Model file for the job. Use its own axes, mm. A direction names the side the tool comes from. Coordinates: 2 decimals unless noted, no trailing zeros. Order: outer loops, then holes, each group sorted by start corner. A loop starts at its lowest first (then second) coordinate and runs counter-clockwise, first axis right, second up. Notation, with made-up numbers: (50.5, 51) -> (59.5, 51) arc R21 cw to (59.5, 87) -> close; hole circle Ø5 at (2.5, -20). An arc over 180 degrees is marked (long way). Return JSON: item names as keys, results as strings. Group by question number.
1) Cut at B-B (z = -102.5). Write the cut outline in (x, y), and give its area (3 significant figures).
2) Flat gauge pins, fed straight in: pin 1 (9.5 mm diameter, centred on y = 172, z = 267.5, fed in from +X); pin 2 (2 mm diameter, centred on x = 152.5, y = 166.5, fed in from -Z); pin 3 (5 mm diameter, centred on y = 247.12, z = -31.83, fed in from -X). Where does each tip first touch, or does it go through?
3) Cut at A-A (x = 2). Write the cut outline in (y, z), and give its area (3 significant figures).
4) Pull direction X, two halves, no side cores. Call faces 5 (the flat face through (150, 101, 328)), 6 (the cylindrical face through (199.014, 138.708, 247.599)), 7 (the flat face through (148, 103, 326)): +X half, -X half, draft (parallel to the pull), parting line (faces both ways), or undercut.
5) Probe line 1 (Y direction, x = 14.5, z = -236.95); line 2 (Y direction, x = 14, z = -237); line 3 (Z direction, x = -135.5, y = 55). List the from-to ranges inside material, lowest first.
6) Which spindle directions (+Z, -Z, +X, -X, +Y, -Y) get a long thin tool onto all of the face, cutting with end or side? Do faces 1 (the flat face through (198, 140, 31)), 2 (the cylindrical face through (-199.01, 231.29, -94.59)), 3 (the flat face through (175, 101, 292.174)), 4 (the flat face through (149.081, 171.234, 320.121)). Say none if no direction does.
from build123d import *

# Parameters (mm, degrees)
BOSS_EXTRUDE1_DEPTH     = 1.5
BOSS_EXTRUDE2_DEPTH     = 280
SKETCH4_W               = 400
SKETCH4_H               = 42.385541564
BOSS_EXTRUDE3_DEPTH     = 2
CUT_EXTRUDE1_DEPTH      = 609.61485268
CUT_EXTRUDE1_DEPTH_BACK = 609.61485268
SKETCH8_R               = 4.39
SKETCH8_R_2             = 2.39
BOSS_EXTRUDE5_DEPTH     = 15
SKETCH10_R              = 3
CUT_EXTRUDE2_DEPTH      = 2
SKETCH5_R               = 2
SKETCH5_R_2             = 10
CUT_EXTRUDE7_DEPTH      = 2
SKETCH21_W              = 300
SKETCH21_H              = 1.5
BOSS_EXTRUDE9_DEPTH     = 10
SKETCH22_W              = 300
SKETCH22_H              = 1.5
BOSS_EXTRUDE10_DEPTH    = 10
BOSS_EXTRUDE11_DEPTH    = 0.75
BOSS_EXTRUDE12_DEPTH    = 0.75
BOSS_EXTRUDE13_DEPTH    = 0.75
BOSS_EXTRUDE14_DEPTH    = 0.75
SKETCH27_W              = 200
SKETCH27_H              = 1.5
BOSS_EXTRUDE15_DEPTH    = 10
BOSS_EXTRUDE16_DEPTH    = 0.75
BOSS_EXTRUDE17_DEPTH    = 0.75
SKETCH30_R              = 24
SKETCH30_R_2            = 1.5
CUT_EXTRUDE8_DEPTH      = 2
SKETCH33_R              = 2
CUT_EXTRUDE9_DEPTH      = 2
SKETCH42_W              = 340
SKETCH42_H              = 12
SKETCH42_R              = 1.6
CUT_EXTRUDE13_DEPTH     = 40


with BuildPart() as part:
    # Sketch1 → Boss-Extrude1 (new body)
    with BuildSketch(Plane(origin=(0, 0, 0), x_dir=(1, 0, 0), z_dir=(0, 1, 0))):
        Polygon((-200, 237.826300096), (200, 237.826300096), (200, -292.173699904), (150, -292.173699904), (150, -362.173699904), (-200, -362.173699904), align=None)
    extrude(amount=BOSS_EXTRUDE1_DEPTH)

    # Sketch2 → Boss-Extrude2 (add)
    with BuildSketch(Plane(origin=(0, 1.5, 0), x_dir=(1, 0, 0), z_dir=(0, 1, 0))):
        Polygon((-200, 237.826300096), (-200, -362.173699904), (150, -362.173699904), (150, -292.173699904), (200, -292.173699904), (200, 237.826300096), align=None)
        Polygon((-198, 235.826300096), (-198, -360.173699904), (148, -360.173699904), (148, -290.173699904), (198, -290.173699904), (198, 235.826300096), align=None, mode=Mode.SUBTRACT)
    extrude(amount=BOSS_EXTRUDE2_DEPTH)

    # Sketch4 → Boss-Extrude3 (add)
    with BuildSketch(Plane(origin=(0, 0, -237.826300096), x_dir=(-1, 0, 0), z_dir=(0, 0, -1))):
        with Locations((0, 213.483316708)):
            Rectangle(SKETCH4_W, SKETCH4_H)
    extrude(amount=-BOSS_EXTRUDE3_DEPTH)

    # Sketch3 → Cut-Extrude1 (cut, two sides: drawn at the far end of the back side and taken through both)
    with BuildSketch(Plane.ZY.offset(200).offset(-CUT_EXTRUDE1_DEPTH_BACK)):
        Polygon((362.173699904, 121.117558148), (227.596852099, 281.5), (362.173699904, 281.5), align=None)
    extrude(amount=CUT_EXTRUDE1_DEPTH + CUT_EXTRUDE1_DEPTH_BACK, mode=Mode.SUBTRACT)

    # Sketch8 → Boss-Extrude5 (add)
    # profile 1 of 2: a face of its own
    with BuildSketch(Plane(origin=(-198, 0, 0), x_dir=(0, 0, -1), z_dir=(1, 0, 0))):
        with Locations((-265.673697326, 172.19919718)):
            Circle(SKETCH8_R)
        with Locations((-265.673697326, 172.19919718)):
            Circle(SKETCH8_R_2, mode=Mode.SUBTRACT)
    # profile 2 of 2: a face of its own
    with BuildSketch(Plane(origin=(-198, 0, 0), x_dir=(0, 0, -1), z_dir=(1, 0, 0))):
        with Locations((-265.173699904, 16.5)):
            Circle(SKETCH8_R)
        with Locations((-265.173699904, 16.5)):
            Circle(SKETCH8_R_2, mode=Mode.SUBTRACT)
    extrude(amount=BOSS_EXTRUDE5_DEPTH)

    # Sketch10 → Cut-Extrude2 (cut)
    with BuildSketch(Plane.ZY.offset(-148)):
        with BuildLine():
            Line((333.923699904, 90.5), (319.923699904, 90.5))
            Line((319.923699904, 90.5), (319.923699904, 87.5))
            Line((319.923699904, 87.5), (315.673699904, 87.5))
            ThreePointArc((315.673699904, 87.5), (304.673699904, 76.5), (315.673699904, 65.5))
            Line((315.673699904, 65.5), (338.173699904, 65.5))
            ThreePointArc((338.173699904, 65.5), (349.173699904, 76.5), (338.173699904, 87.5))
            Line((338.173699904, 87.5), (333.923699904, 87.5))
            Line((333.923699904, 87.5), (333.923699904, 90.5))
        make_face()
        with Locations((300.973699904, 103.45)):
            Circle(SKETCH10_R)
        with Locations((352.873699904, 103.45)):
            Circle(SKETCH10_R)
        with Locations((300.973699904, 49.55)):
            Circle(SKETCH10_R)
        with Locations((352.873699904, 49.55)):
            Circle(SKETCH10_R)
    extrude(amount=-CUT_EXTRUDE2_DEPTH, mode=Mode.SUBTRACT)

    # Sketch5 → Cut-Extrude7 (cut)
    with BuildSketch(Plane.ZY.offset(200)):
        with Locations((-115.826300096, 247.120648807)):
            Circle(SKETCH5_R)
        with Locations((-116.326300096, 223.125857706)):
            Circle(SKETCH5_R)
        with Locations((-91.826300096, 223.120648807)):
            Circle(SKETCH5_R)
        with Locations((-91.826300096, 247.120648807)):
            Circle(SKETCH5_R)
        with Locations((-103.826300096, 235.120648807)):
            Circle(SKETCH5_R_2)
        with Locations((-55.826300096, 247.120648807)):
            Circle(SKETCH5_R)
        with Locations((-56.326300096, 223.125857706)):
            Circle(SKETCH5_R)
        with Locations((-31.826300096, 223.120648807)):
            Circle(SKETCH5_R)
        with Locations((-31.826300096, 247.120648807)):
            Circle(SKETCH5_R)
        with Locations((-43.826300096, 235.120648807)):
            Circle(SKETCH5_R_2)
        with Locations((4.173699904, 247.120648807)):
            Circle(SKETCH5_R)
        with Locations((3.673699904, 223.125857706)):
            Circle(SKETCH5_R)
        with Locations((28.173699904, 223.120648807)):
            Circle(SKETCH5_R)
        with Locations((28.173699904, 247.120648807)):
            Circle(SKETCH5_R)
        with Locations((16.173699904, 235.120648807)):
            Circle(SKETCH5_R_2)
        with Locations((64.173699904, 247.120648807)):
            Circle(SKETCH5_R)
        with Locations((63.673699904, 223.125857706)):
            Circle(SKETCH5_R)
        with Locations((88.173699904, 223.120648807)):
            Circle(SKETCH5_R)
        with Locations((88.173699904, 247.120648807)):
            Circle(SKETCH5_R)
        with Locations((76.173699904, 235.120648807)):
            Circle(SKETCH5_R_2)
    extrude(amount=-CUT_EXTRUDE7_DEPTH, mode=Mode.SUBTRACT)

    # Sketch21 → Boss-Extrude9 (add)
    with BuildSketch(Plane(origin=(0, 0, -237.826300096), x_dir=(-1, 0, 0), z_dir=(0, 0, -1))):
        with Locations((0, 270.75)):
            Rectangle(SKETCH21_W, SKETCH21_H)
    extrude(amount=BOSS_EXTRUDE9_DEPTH)

    # Sketch22 → Boss-Extrude10 (add)
    with BuildSketch(Plane.ZY.offset(200)):
        with Locations((-7.826300096, 270.75)):
            Rectangle(SKETCH22_W, SKETCH22_H)
    boss_extrude10 = extrude(amount=BOSS_EXTRUDE10_DEPTH)

    # Sketch23 → Boss-Extrude11 (add, symmetric)
    with BuildSketch(Plane(origin=(0, 0, -77.826300096), x_dir=(-1, 0, 0), z_dir=(0, 0, -1))):
        Polygon((210, 270), (200, 270), (200, 260), align=None)
    boss_extrude11 = extrude(amount=BOSS_EXTRUDE11_DEPTH, both=True)

    # Sketch24 → Boss-Extrude12 (add, symmetric)
    with BuildSketch(Plane.XY.offset(52.173699904)):
        Polygon((-210, 270), (-200, 260), (-200, 270), align=None)
    boss_extrude12 = extrude(amount=BOSS_EXTRUDE12_DEPTH, both=True)

    # Sketch25 → Boss-Extrude13 (add, symmetric)
    with BuildSketch(Plane(origin=(100, 0, 0), x_dir=(0, 0, -1), z_dir=(1, 0, 0))):
        Polygon((247.826300096, 270), (237.826300096, 270), (237.826300096, 260), align=None)
    extrude(amount=BOSS_EXTRUDE13_DEPTH, both=True)

    # Sketch26 → Boss-Extrude14 (add, symmetric)
    with BuildSketch(Plane.ZY.offset(100)):
        Polygon((-247.826300096, 270), (-237.826300096, 260), (-237.826300096, 270), align=None)
    extrude(amount=BOSS_EXTRUDE14_DEPTH, both=True)

    # Mirror1: Boss-Extrude10, Boss-Extrude11, Boss-Extrude12 across plane
    add(boss_extrude10.mirror(Plane(origin=(0, 0, 0), x_dir=(0, 0, 1), z_dir=(1, 0, 0))))
    add(boss_extrude11.mirror(Plane(origin=(0, 0, 0), x_dir=(0, 0, 1), z_dir=(1, 0, 0))))
    add(boss_extrude12.mirror(Plane(origin=(0, 0, 0), x_dir=(0, 0, 1), z_dir=(1, 0, 0))))

    # Sketch27 → Boss-Extrude15 (add)
    with BuildSketch(Plane.XY.offset(362.173699904)):
        with Locations((-25, 110.367558148)):
            Rectangle(SKETCH27_W, SKETCH27_H)
    extrude(amount=BOSS_EXTRUDE15_DEPTH)

    # Sketch28 → Boss-Extrude16 (add, symmetric)
    with BuildSketch(Plane.ZY.offset(95)):
        Polygon((372.173699904, 109.617558148), (362.173699904, 109.617558148), (362.173699904, 99.617558148), align=None)
    extrude(amount=BOSS_EXTRUDE16_DEPTH, both=True)

    # Sketch29 → Boss-Extrude17 (add, symmetric)
    with BuildSketch(Plane(origin=(45, 0, 0), x_dir=(0, 0, -1), z_dir=(1, 0, 0))):
        Polygon((-372.173699904, 109.617558148), (-362.173699904, 99.617558148), (-362.173699904, 109.617558148), align=None)
    extrude(amount=BOSS_EXTRUDE17_DEPTH, both=True)

    # Sketch30 → Cut-Extrude8 (cut)
    with BuildSketch(Plane(origin=(200, 0, 0), x_dir=(0, 0, -1), z_dir=(1, 0, 0))):
        with Locations((-258.673699904, 160)):
            Circle(SKETCH30_R)
        with Locations((-284.673699904, 150)):
            Circle(SKETCH30_R_2)
        with Locations((-232.673699904, 150)):
            Circle(SKETCH30_R_2)
    extrude(amount=-CUT_EXTRUDE8_DEPTH, mode=Mode.SUBTRACT)

    # Sketch33 → Cut-Extrude9 (cut)
    with BuildSketch(Plane.ZY.offset(200)):
        with Locations((-180.626300096, 147.77)):
            Circle(SKETCH33_R)
        with Locations((-180.626300096, 28.39)):
            Circle(SKETCH33_R)
        with Locations((-8.926300096, 147.77)):
            Circle(SKETCH33_R)
        with Locations((-8.926300096, 28.39)):
            Circle(SKETCH33_R)
        with Locations((162.773699904, 147.77)):
            Circle(SKETCH33_R)
        with Locations((162.773699904, 28.39)):
            Circle(SKETCH33_R)
    extrude(amount=-CUT_EXTRUDE9_DEPTH, mode=Mode.SUBTRACT)

    # Sketch42 → Cut-Extrude13 (cut)
    with BuildSketch(Plane.XY.offset(-235.826300096)):
        with Locations((0, 225.5)):
            Rectangle(SKETCH42_W, SKETCH42_H)
        with Locations((-120.5, 240)):
            Circle(SKETCH42_R)
        with Locations((-149.5, 211)):
            Circle(SKETCH42_R)
        with Locations((-75.5, 240)):
            Circle(SKETCH42_R)
        with Locations((-104.5, 211)):
            Circle(SKETCH42_R)
        with Locations((-30.5, 240)):
            Circle(SKETCH42_R)
        with Locations((-59.5, 211)):
            Circle(SKETCH42_R)
        with Locations((14.5, 240)):
            Circle(SKETCH42_R)
        with Locations((-14.5, 211)):
            Circle(SKETCH42_R)
        with Locations((59.5, 240)):
            Circle(SKETCH42_R)
        with Locations((30.5, 211)):
            Circle(SKETCH42_R)
        with Locations((104.5, 240)):
            Circle(SKETCH42_R)
        with Locations((75.5, 211)):
            Circle(SKETCH42_R)
        with Locations((149.5, 240)):
            Circle(SKETCH42_R)
        with Locations((120.5, 211)):
            Circle(SKETCH42_R)
    extrude(amount=-CUT_EXTRUDE13_DEPTH, mode=Mode.SUBTRACT)


solid = part.part
Answers below:
{
 "1": {"outline": "(-210, 270) -> (-200, 270) -> (-200, 245.03) -> (-198, 245.03) -> (-198, 281.5) -> (-200, 281.5) -> (-200, 271.5) -> (-210, 271.5) -> close; (-200, 0) -> (200, 0) -> (200, 270) -> (210, 270) -> (210, 271.5) -> (200, 271.5) -> (200, 281.5) -> (198, 281.5) -> (198, 1.5) -> (-198, 1.5) -> (-198, 225.21) -> (-200, 225.21) -> close", "area": "1,710 mm^2"},
 "2": {"pin 1": "stops at x = -183", "pin 2": "stops at z = -237.83", "pin 3": "stops at x = -200"},
 "3": {"outline": "(0, -237.83) -> (219.5, -237.83) -> (219.5, -235.83) -> (1.5, -235.83) -> (1.5, 360.17) -> (123.5, 360.17) -> (121.12, 362.17) -> (111.12, 362.17) -> (111.12, 372.17) -> (109.62, 372.17) -> (109.62, 362.17) -> (0, 362.17) -> close; (231.5, -237.83) -> (270, -237.83) -> (270, -247.83) -> (271.5, -247.83) -> (271.5, -237.83) -> (281.5, -237.83) -> (281.5, -235.83) -> (231.5, -235.83) -> close", "area": "1,710 mm^2"},
 "4": {"face 5": "+X half", "face 6": "draft", "face 7": "undercut"},
 "5": {"line 1": "y = 0 to 219.5, 231.5 to 238.4, 241.6 to 281.5", "line 2": "y = 0 to 219.5, 231.5 to 238.48, 241.52 to 281.5", "line 3": "z = -237.83 to -235.83, 360.17 to 362.17"},
 "6": {"face 1": "+Y", "face 2": "-X", "face 3": "+Z, +X, +Y, -Y", "face 4": "+Z, +X, -X, +Y"}
}
